Here's how the part is built. I have some questions about the finished solid (model axes, mm). A direction names the side the tool comes from. Round coordinates to 2 decimals unless told otherwise and drop trailing zeros. Order: outer loops, then holes, each group sorted by start corner. A loop starts at its lowest first (then second) coordinate and runs counter-clockwise, first axis right, second up.
```python
from build123d import *


with BuildPart() as part:
    # Sketch1 → Revolve1 (revolve)
    with BuildSketch(Plane(origin=(0, 0, 0), x_dir=(0, 0, -1), z_dir=(1, 0, 0)), mode=Mode.PRIVATE) as revolve1_sk:
        with BuildLine():
            ThreePointArc((0.7, 5.6), (0, 4.9), (-0.7, 5.6))
            Line((-0.7, 5.6), (-0.7, 6))
            Line((-0.7, 6), (-1.5, 6))
            Line((-1.5, 6), (-1.5, 1.5))
            Line((-1.5, 1.5), (1.5, 1.5))
            Line((1.5, 1.5), (1.5, 6))
            Line((1.5, 6), (0.7, 6))
            Line((0.7, 6), (0.7, 5.6))
        make_face()
    revolve(revolve1_sk.sketch.rotate(Axis((0, 0, 1.5), (0, 0, -1)), 90), axis=Axis((0, 0, 1.5), (0, 0, -1)))


solid = part.part
```
1. If we section it at C-C, the plane z = -1.2: Write out the boundary of the cut face in (x, y).
Evaluation:
outline: circle Ø12 at (0, 0); hole circle Ø3 at (0, 0)
2. If we mould it in two halves opening along Y, with no side actions, what happens to faces 1 (the cylindrical face through (5.723, -1.802, 1.106)), 2 (the flat face through (1.2, 1.2, 1.5)), 3 (the cylindrical face through (1.43, -0.45, -0.02))? For each: released by +Y, released by -Y, zero draft, split by the parting line, or undercut.
Evaluation:
face 1: split by the parting line
face 2: zero draft
face 3: undercut
3. If we section it at D-D, the plane z = -0.1: Write out the boundary of the cut face in (x, y).
Evaluation:
outline: circle Ø9.81 at (0, 0); hole circle Ø3 at (0, 0)
4. I'm going to push flat-ended pins straight in: P1, Ø1.5, axis at y = 3, z = 0.5, coming from the -X side; P2, Ø1, axis at y = 2, z = 1, coming from the +X side. Where does each tip first touch, or does it pass through?
Evaluation:
P1: stops at x = -5.55
P2: stops at x = 5.81
5. If we section it at A-A, the plane y = 0: Write out the boundary of the cut face in (x, z).
Evaluation:
outline: (-6, -1.5) - (-1.5, -1.5) - (-1.5, 1.5) - (-6, 1.5) - (-6, 0.7) - (-5.6, 0.7) arc R0.7 cw to (-5.6, -0.7) - (-6, -0.7) - close; (1.5, -1.5) - (6, -1.5) - (6, -0.7) - (5.6, -0.7) arc R0.7 cw to (5.6, 0.7) - (6, 0.7) - (6, 1.5) - (1.5, 1.5) - close
6. On a 3-axis mill with a long thin cutter (end or side, diameter ignored), from which of +Z, -Z, +X, -X, +Y, -Y can I reach the whole of each face in a straight line? I mean faces 4 (the flat face through (5, -3, 0.7)), 5 (the flat face through (-1.2, 1.2, -1.5)). Say none if no direction works.
Evaluation:
face 4: none
face 5: -Z, +X, -X, +Y, -Y
7. I need wall thicknesses on probe 1 along Z at (x, y) = (0, 5.75); probe 2 along Z at (x, y) = (0.75, -5); probe 3 along X at (y, z) = (1.25, -0.95). Which ranges of each line are inside material? Lowest first, please.
Evaluation:
probe 1: z = -1.5 to -0.7, 0.7 to 1.5
probe 2: z = -1.5 to -0.44, 0.44 to 1.5
probe 3: x = -5.87 to -0.83, 0.83 to 5.87
